Verification items for the finished model (mm, model axes). A direction names the side the tool comes from. Coordinates: 2 decimals unless noted, no trailing zeros. Order: outer loops, then holes, each group sorted by start corner. A loop starts at its lowest first (then second) coordinate and runs counter-clockwise, first axis right, second up. Notation, with made-up numbers: M -19,79.25 L 20,79.25 A16 cw 20,93.25 Z; hole C 12,69 d7. An arc over 180 degrees is marked long. Return JSON: item names as keys, results as strings. Group by question number.
Q1. Section check D-D, the plane x = -26.5. Enter the section's corners in (y, z).
Q2. Section check A-A, the plane y = 10.5. Enter the section's corners in (x, z).
Q3. Mould release check, pull along X, two halves, no side actions. Record for faces 1 (the face through (30, 7, 3)), 2 (the face through (-43.189, 10, 1)), 3 (the face through (16, 10, 21.594)): pulls with the +X half, pulls with the -X half, needs draft (parallel to the pull), parting line crosses it, or undercut.
Q4. Access from +Z, -Z, +X, -X, +Y, -Y to the whole of each face (thin tool, end or side, straight path). Record for faces 4 (the face through (49.81, 10.63, 0.22)), 5 (the face through (9, 7, 3)).
Q5. Section check B-B, the plane z = -17. Enter the section's corners in (x, y).
Q6. Go/stop test with flat-tipped pins: pin 1 Ø9.5 at (x, y) = (46.81, 10.5) entering from -Z; pin 2 Ø10 at (x, z) = (29.5, -1) entering from +Y. Record where each tip stops, or that it passes through.
Q7. Thickness scan on probe 1 along Y at (x, z) = (62.5, 7.5); probe 2 along X at (y, z) = (8, 17.5); probe 3 along X at (y, z) = (8.5, -2). Record the ranges inside material, lowest first.
Q8. Section check C-C, the plane y = 39. Enter the section's corners in (x, z).
from build123d import *

# Parameters (mm, degrees)
SKETCH1_W           = 120
SKETCH1_H           = 42.16
BOSS_EXTRUDE1_DEPTH = 21
CUT_EXTRUDE1_DEPTH  = 14
SKETCH3_R           = 3.25
CUT_EXTRUDE2_DEPTH  = 82.007752785
FILLET1_R           = 1
FILLET2_R           = 0.5
BOSS_EXTRUDE2_DEPTH = 40
SKETCH19_R          = 3
CUT_EXTRUDE3_DEPTH  = 107.763288693


with BuildPart() as part:
    # Sketch1 → Boss-Extrude1 (new body)
    with BuildSketch(Plane(origin=(0, 0, 0), x_dir=(1, 0, 0), z_dir=(0, 1, 0))):
        with Locations((16.811029237, -0.514485382)):
            Rectangle(SKETCH1_W, SKETCH1_H)
    extrude(amount=BOSS_EXTRUDE1_DEPTH)

    # Sketch2 → Cut-Extrude1 (cut)
    with BuildSketch(Plane(origin=(0, 21, 0), x_dir=(1, 0, 0), z_dir=(0, 1, 0))):
        with BuildLine():
            ThreePointArc((27.061029237, 5.735514618), (20.811029237, -0.514485382), (27.061029237, -6.764485382))
            Line((27.061029237, -6.764485382), (27.061029237, 5.735514618))
        make_face()
        with BuildLine():
            Line((27.061029237, 5.735514618), (27.061029237, -6.764485382))
            ThreePointArc((27.061029237, -6.764485382), (31.480446619, -4.933902764), (33.311029237, -0.514485382))
            ThreePointArc((33.311029237, -0.514485382), (31.480446619, 3.904932001), (27.061029237, 5.735514618))
        make_face()
        with BuildLine():
            ThreePointArc((6.561029237, 5.735514618), (0.311029237, -0.514485382), (6.561029237, -6.764485382))
            Line((6.561029237, -6.764485382), (6.561029237, 5.735514618))
        make_face()
        with BuildLine():
            Line((6.561029237, 5.735514618), (6.561029237, -6.764485382))
            ThreePointArc((6.561029237, -6.764485382), (10.980446619, -4.933902764), (12.811029237, -0.514485382))
            ThreePointArc((12.811029237, -0.514485382), (10.980446619, 3.904932001), (6.561029237, 5.735514618))
        make_face()
    extrude(amount=-CUT_EXTRUDE1_DEPTH, mode=Mode.SUBTRACT)

    # Sketch3 → Cut-Extrude2 (cut, through all)
    with BuildSketch(Plane(origin=(0, 7, 0), x_dir=(1, 0, 0), z_dir=(0, 1, 0))):
        with Locations(Location((27.061029237, -0.514485382, 0), (0, 0, 270))):
            Circle(SKETCH3_R)
        with Locations(Location((6.561029237, -0.514485382, 0), (0, 0, 270))):
            Circle(SKETCH3_R)
    extrude(amount=-CUT_EXTRUDE2_DEPTH, mode=Mode.SUBTRACT)

    # Fillet1
    fillet1_edges = [part.edges().sort_by_distance(p)[0] for p in [
        (27.061029237, 21, 6.764485382),
        (6.561029237, 21, 6.764485382),
    ]]
    fillet(fillet1_edges, radius=FILLET1_R)

    # Fillet2
    fillet2_edges = [part.edges().sort_by_distance(p)[0] for p in [
        (27.061029237, 0, -2.735514618),
        (6.561029237, 0, -2.735514618),
    ]]
    fillet(fillet2_edges, radius=FILLET2_R)

    # Sketch4 → Boss-Extrude2 (add)
    with BuildSketch(Plane(origin=(0, 21, 0), x_dir=(1, 0, 0), z_dir=(0, 1, 0))):
        with BuildLine():
            ThreePointArc((52.461029237, 3.485514618), (48.461029237, -0.514485382), (52.461029237, -4.514485382))
            Line((52.461029237, -4.514485382), (52.461029237, 3.485514618))
        make_face()
        with BuildLine():
            Line((52.461029237, 3.485514618), (52.461029237, -4.514485382))
            ThreePointArc((52.461029237, -4.514485382), (55.289456362, -3.342912506), (56.461029237, -0.514485382))
            ThreePointArc((56.461029237, -0.514485382), (55.289456362, 2.313941743), (52.461029237, 3.485514618))
        make_face()
        with BuildLine():
            ThreePointArc((-18.838970763, 3.485514618), (-22.838970763, -0.514485382), (-18.838970763, -4.514485382))
            Line((-18.838970763, -4.514485382), (-18.838970763, 3.485514618))
        make_face()
        with BuildLine():
            Line((-18.838970763, 3.485514618), (-18.838970763, -4.514485382))
            ThreePointArc((-18.838970763, -4.514485382), (-16.010543638, -3.342912506), (-14.838970763, -0.514485382))
            ThreePointArc((-14.838970763, -0.514485382), (-16.010543638, 2.313941743), (-18.838970763, 3.485514618))
        make_face()
    extrude(amount=BOSS_EXTRUDE2_DEPTH)

    # Sketch19 → Cut-Extrude3 (cut, through all)
    with BuildSketch(Plane(origin=(0, 0, -20.565514618), x_dir=(-1, 0, 0), z_dir=(0, 0, -1))):
        with Locations((13.188970763, 10.5)):
            Circle(SKETCH19_R)
        with Locations((-46.811029237, 10.5)):
            Circle(SKETCH19_R)
    extrude(amount=-CUT_EXTRUDE3_DEPTH, mode=Mode.SUBTRACT)


solid = part.part
Numbers:
{
 "1": {"outline": "M 0,-20.57 L 21,-20.57 L 21,21.59 L 0,21.59 Z"},
 "2": {"outline": "M -43.19,-20.57 L -16.19,-20.57 L -16.19,21.59 L -43.19,21.59 Z; M -10.19,-20.57 L 43.81,-20.57 L 43.81,21.59 L -10.19,21.59 Z; M 49.81,-20.57 L 76.81,-20.57 L 76.81,21.59 L 49.81,21.59 Z; hole C 6.56,0.51 d12.5; hole C 27.06,0.51 d12.5"},
 "3": {"face 1": "undercut", "face 2": "pulls with the -X half", "face 3": "needs draft"},
 "4": {"face 4": "+Z, -Z", "face 5": "+Y"},
 "5": {"outline": "M -43.19,0 L 76.81,0 L 76.81,21 L -43.19,21 Z; hole C -13.19,10.5 d6; hole C 46.81,10.5 d6"},
 "6": {"pin 1": "stops at z = -20.57", "pin 2": "stops at y = 21"},
 "7": {"probe 1": "y = 0 to 21", "probe 2": "x = -43.19 to -14.85, -11.53 to 45.15, 48.47 to 76.81", "probe 3": "x = -43.19 to -15.43, -10.95 to 0.84, 12.28 to 21.34, 32.78 to 44.57, 49.05 to 76.81"},
 "8": {"outline": "C -18.84,0.51 d8; C 52.46,0.51 d8"}
}
